The listing builds one solid part. Answer for the finished solid, in the listing's coordinates (mm). Face numbers are marked on the shaded views. A direction names the side the tool comes from. Give positions to 0.01 mm unless a question says otherwise; leave off trailing zeros. Order: outer loops, then holes, each group sorted by start corner. A loop starts at its lowest first (then second) coordinate and runs counter-clockwise, first axis right, second up. Notation, with made-up numbers: (41, 53) - (60, 53) arc R20 cw to (60, 59) - close; hole circle Ø3 at (-37, 24.25). An arc over 180 degrees is marked (long way). Write each question's results on one line, items separated by ' | '. Start each with the question number.
1. Section B-B (y = -5.75) is taken. Give the vertices of the cut face in (x, z).
2. Determine the mould class of the marked faces 6, 7, 8 and 9 for opening direction Z: released by +Z, released by -Z, zero draft, split by the parting line, or undercut.
3. Section C-C (y = 8.5) is taken. Give the vertices of the cut face in (x, z), and give its area (3 significant figures).
4. Flat-ended cylindrical pins translate along their axes: pin 1 (4 mm diameter, centred on x = 0, y = 16.5, fed in from -Z); pin 2 (4 mm diameter, centred on x = -10.5, y = 18.5, fed in from -Z); pin 3 (7.5 mm diameter, centred on x = -3.5, y = 19, fed in from +Z); pin 4 (4.5 mm diameter, centred on x = -4.5, z = 0, fed in from +Y). Find the tip coordinate at first contact, or state that the pin passes through.
5. Find the intervals of material crossed by L1, parallel to Z at x = 3, y = -9; L2, parallel to Y at x = 0, z = -16.85; L3, parallel to X at y = 16.5, z = 3, in increasing order.
6. Section D-D (x = -7.5) is taken. Give the vertices of the cut face in (y, z), and give its area (3 significant figures).
7. Which of the six approach directions +Z, -Z, +X, -X, +Y, -Y give full straight-line access (tool end or side, diameter ignored) to the marked faces 1, 2, 3, 4 and 5?
Autodesk Inventor part; units mm, degrees
ref_plane "YZ Plane" through (0, 0, 0) normal (1, 0, 0) x (0, 1, 0)
ref_plane "XZ Plane" through (0, 0, 0) normal (0, 1, 0) x (-1, 0, 0)
ref_plane "XY Plane" through (0, 0, 0) normal (0, 0, 1) x (1, 0, 0)
sketch "Sketch2" plane through (0, 0, 0) normal (1, 0, 0) x (0, 1, 0)
  line L0 (0, -12.532) -> (0, 12.468)
  line L1 (0, 12.468) -> (3, 12.468)
  line L2 (3, -12.532) -> (3, 12.468)
  line L3 (0, -12.532) -> (3, -12.532)
  line L4 (-17, -12.532) -> (3, -12.532)
  line L5 (3, -12.532) -> (3, -15.532)
  line L6 (-17, -15.532) -> (3, -15.532)
  line L7 (-17, -12.532) -> (-17, -15.532)
  line L8 (3.5, -13.032) -> (3.5, -0.032)
  line L9 (-11.5, -16.032) -> (3.5, -16.032)
  line L10 (3.5, -13.032) -> (3.5, -16.032)
  line L11 (-11.5, -19.032) -> (6.5, -19.032)
  line L12 (3.5, -0.032) -> (6.5, -0.032) construction
  line L13 (-11.5, -16.032) -> (-11.5, -19.032)
  line L14 (6.5, -2.032) -> (31.5, -2.032)
  line L15 (31.5, -2.032) -> (31.5, -5.032)
  line L16 (31.5, -5.032) -> (6.5, -5.032)
  line L17 (3.5, 12.968) -> (3.5, -0.032)
  line L18 (-11.5, 15.968) -> (3.5, 15.968)
  line L19 (3.5, 12.968) -> (3.5, 15.968)
  line L20 (-11.5, 18.968) -> (6.5, 18.968)
  line L21 (-11.5, 15.968) -> (-11.5, 18.968)
  line L22 (6.5, 1.968) -> (31.5, 1.968)
  line L23 (31.5, 1.968) -> (31.5, 4.968)
  line L24 (31.5, 4.968) -> (6.5, 4.968)
  line L25 (3, 12.468) -> (-17, 12.468)
  line L26 (-17, 12.468) -> (-17, 15.468)
  line L27 (3, 15.468) -> (-17, 15.468)
  line L28 (3, 12.468) -> (3, 15.468)
  line L29 (6.5, 18.968) -> (6.5, 4.968)
  line L30 (6.5, 1.968) -> (6.5, -0.032)
  line L31 (6.5, -19.032) -> (6.5, -5.032)
  line L32 (6.5, -2.032) -> (6.5, -0.032)
  point P0 (0, 0)
  dimension "d0" = 0.5
  dimension "d1" = 0.5
  dimension "d3" = 15
  dimension "d4" = 3
  dimension "d5" = 19
  dimension "d7" = 25
  dimension "d8" = 2
  dimension "d9" = 3
  dimension "d11" = 3.5
extrude "Extrusion1" add sketch "Sketch2" along normal blind 15 and the other way blind 15 contours L8 L17 L19 L18 L21 L20 L29 L24 L23 L22 L30 L32 L14 L15 L16 L31 L11 L13 L9 L10
fillet "Fillet1" radius 15 4 edges at (-15, 31.5, -3.532) (-15, 31.5, 3.468) (15, 31.5, -3.532) (15, 31.5, 3.468)
sketch "Sketch3" plane through (15, 6.5, -19.032) normal (0, 0, -1) x (-1, 0, 0)
  line L0 (-110, -6.5) -> (140, -6.5)
  line L1 (0, -18) -> (30, -18)
  line L2 (0, -18) -> (0, 0)
  line L3 (30, 0) -> (30, -18)
  point P0 (15, -6.5)
  point P1 (15, -12.25)
  dimension "d17" = 5.75
  dimension "d18" = 15
hole "Hole1" at (0, -5.75, -19.032) direction (0, 0, 1) diameter 5 depth 300 tip angle 118
sketch "Sketch4" plane through (15, 6.5, -5.032) normal (0, 0, -1) x (-1, 0, 0)
  arc A0 (30, 10) -> (0, 10) centre (15, 10) ccw
  point P0 (15, -6.5)
hole "Hole2" at (0, 16.5, -5.032) direction (0, 0, 1) diameter 5 depth 300 tip angle 118
properties part number "Sujetador_Carril"
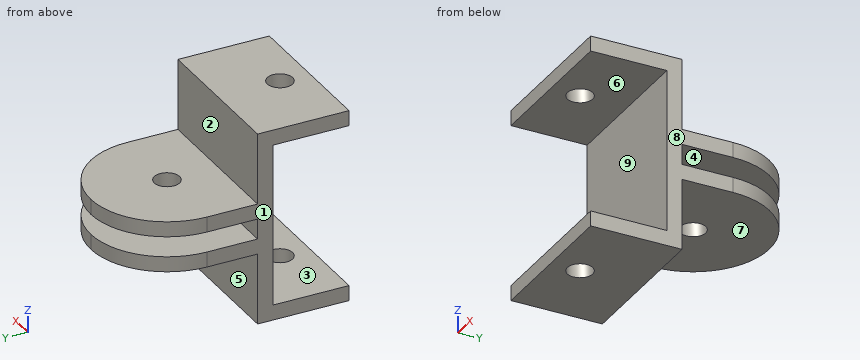
Reported:
1) outline: (-15, -19.03) - (-2.5, -19.03) - (-2.5, -16.03) - (-15, -16.03) - close; (-15, 15.97) - (-2.5, 15.97) - (-2.5, 18.97) - (-15, 18.97) - close; (2.5, -19.03) - (15, -19.03) - (15, -16.03) - (2.5, -16.03) - close; (2.5, 15.97) - (15, 15.97) - (15, 18.97) - (2.5, 18.97) - close
2) face 6: undercut | face 7: released by -Z | face 8: zero draft | face 9: undercut
3) outline: (-15, -5.03) - (15, -5.03) - (15, -2.03) - (-15, -2.03) - close; (-15, 1.97) - (15, 1.97) - (15, 4.97) - (-15, 4.97) - close | area: 180 mm²
4) pin 1: through | pin 2: z = -5.03 | pin 3: z = 4.97 | pin 4: y = 31.11
5) L1: -19.03 to -16.03, 15.97 to 18.97 | L2: -11.5 to -8.25, -3.25 to 6.5 | L3: -15 to -2.5, 2.5 to 15
6) outline: (-11.5, -19.03) - (6.5, -19.03) - (6.5, -5.03) - (29.49, -5.03) - (29.49, -2.03) - (6.5, -2.03) - (6.5, 1.97) - (29.49, 1.97) - (29.49, 4.97) - (6.5, 4.97) - (6.5, 18.97) - (-11.5, 18.97) - (-11.5, 15.97) - (3.5, 15.97) - (3.5, -16.03) - (-11.5, -16.03) - close | area: 342 mm²
7) face 1: +Z, -Z, -X, +Y, -Y | face 2: +Z, +X, -X, +Y | face 3: +X, -X, -Y | face 4: +X, -X, +Y | face 5: -Z, +X, -X, +Y
